Verification items for the finished model (mm, model axes). A direction names the side the tool comes from. Round coordinates to 2 decimals unless told otherwise and drop trailing zeros. Order: outer loops, then holes, each group sorted by start corner. A loop starts at its lowest first (then second) coordinate and runs counter-clockwise, first axis right, second up. Notation, with made-up numbers: M 50,-16.75 L 58,-16.75 A14 cw 58,5.25 Z; hole C -9.75,-23 d6. An arc over 180 degrees is marked long. Write item = value, one per line. Start each with the question number.
from build123d import *

# Parameters (mm, degrees)
F0_W     = 67.1
F0_H     = 120
F1_DEPTH = 4
F2_R     = 5
F3_T     = -1


with BuildPart() as f1:
    # F0 (on Front) → F1 (new body)
    with BuildSketch(Plane.XZ):
        Rectangle(F0_W, F0_H)
    extrude(amount=F1_DEPTH)

    # F2
    f2_edges = [f1.edges().sort_by_distance(p)[0] for p in [
        (33.55, -2, -60),
        (-33.55, -2, -60),
    ]]
    fillet(f2_edges, radius=F2_R)

    # F3
    f3_openings = [f1.faces().sort_by_distance(p)[0] for p in [
        (0, -2, 60),
    ]]
    offset(amount=F3_T, openings=f3_openings)


solid = f1.part
1) Access from +Z, -Z, +X, -X, +Y, -Y to the whole of each face (thin tool, end or side, straight path). Record for faces 1 (the flat face through (33.55, -2, 2)), 2 (the cylindrical face through (-31.409, -2.014, -57.797)).
2) Gauge pin test, flat end, axial feed: P1, Ø1.5, axis at x = -11.5, z = 29, coming from the +Y side. Record the tip position at first contact, or that the pin passes through.
3) Scan lines: probe 1 along X at (y, z) = (-2.95, 10); probe 2 along Y at (x, z) = (6.5, -23); probe 3 along Z at (x, y) = (-2, -2). Record each from-to range of solid material in increasing order.
4) Cross-section at A-A, the plane z = -32. Enter the section's corners in (x, y), then the cut area to 3 significant figures.
5) Release check for a two-part mould opening along Y. For faces 3 (the flat face through (0, -3, 1)), 4 (the flat face through (0, 0, 1)), 5 (the cylindrical face through (-32.12, -2.03, -58.5)) record: pulls with the +Y half, pulls with the -Y half, needs draft (parallel to the pull), parting line crosses it, or undercut.
6) Cross-section at C-C, the plane y = -2. Enter the section's corners in (x, z), then the cut area to 3 significant figures.
7) Cross-section at B-B, the plane x = 25.5. Enter the section's corners in (y, z).
Geometry results:
q1.face_1 = +Z, -Z, +X, +Y, -Y
q1.face_2 = +Z
q2.P1 = 0
q3.probe_1 = -33.55 to -32.55, 32.55 to 33.55
q3.probe_2 = -4 to -3, -1 to 0
q3.probe_3 = -60 to -59
q4.outline = M -33.55,-4 L 33.55,-4 L 33.55,0 L -33.55,0 Z; hole M -32.55,-3 L 32.55,-3 L 32.55,-1 L -32.55,-1 Z
q4.area = 138 mm^2
q5.face_3 = undercut
q5.face_4 = pulls with the +Y half
q5.face_5 = needs draft
q6.outline = M -33.55,-55 A5 ccw -28.55,-60 L 28.55,-60 A5 ccw 33.55,-55 L 33.55,60 L 32.55,60 L 32.55,-55 A4 cw 28.55,-59 L -28.55,-59 A4 cw -32.55,-55 L -32.55,60 L -33.55,60 Z
q6.area = 301 mm^2
q7.outline = M -4,-60 L 0,-60 L 0,60 L -1,60 L -1,-59 L -3,-59 L -3,60 L -4,60 Z
